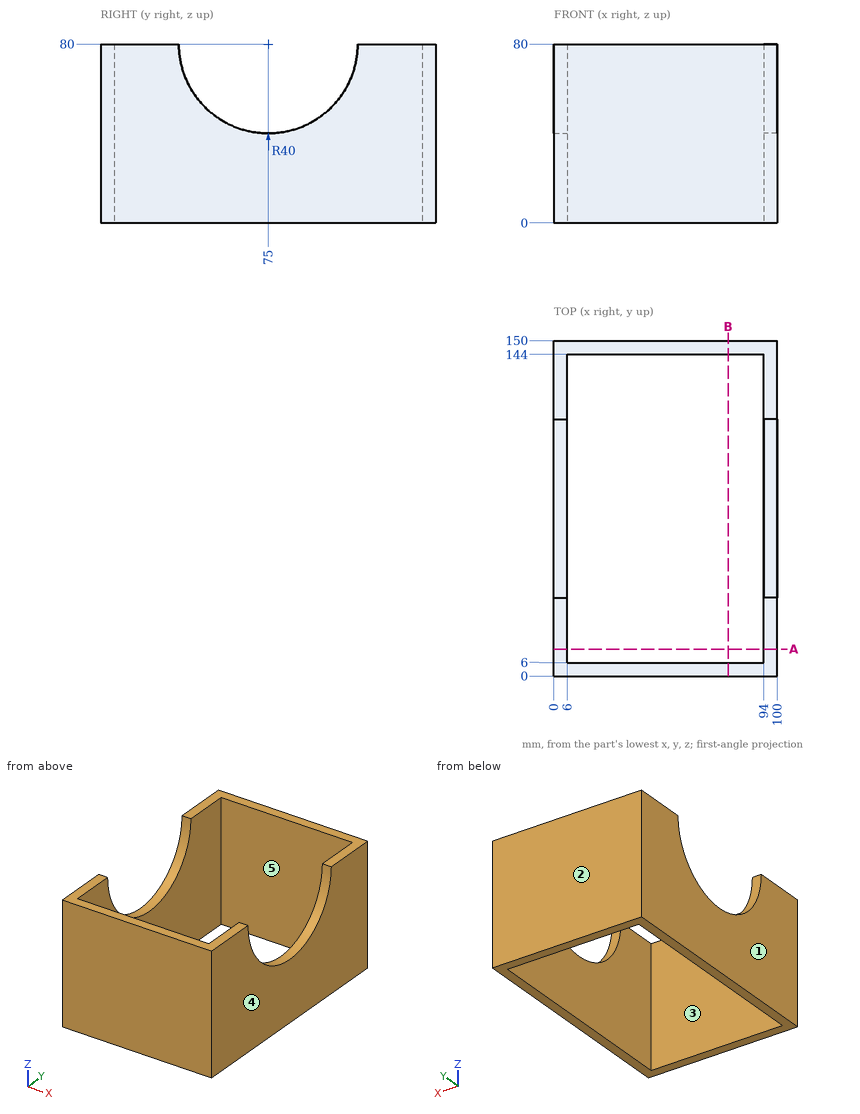
Job drawing, mm, ordinate dimensions from the low corner. One solid piece. A direction names the side the tool comes from. Coordinates: 2 decimals unless noted, no trailing zeros. Loops run counter-clockwise (first coordinate to the right, second up) from the corner with the lowest first, then second, coordinate; pieces in that order, holes last. Notation, with made-up numbers: (-23.75, 2) - (18.25, 2) arc R22 ccw to (18.25, 25) - close; hole circle Ø10 at (26, 73). An arc over 180 degrees is marked (long way). Write item = value, one per line. Start each with the question number.
Q1. Which spindle directions (+Z, -Z, +X, -X, +Y, -Y) get a long thin tool onto all of the face, cutting with end or side? Do the marked faces 4 and 5. Say none if no direction does.
Q2. Drill centre lines: L1, parallel to Y at x = 63.5, z = 9; L2, parallel to X at y = 140.5, z = 11.5. Where is each one in solid material? Low to high.
Q3. Flat gauge pin, fed straight in: pin 1 Ø12 at (x, z) = (43, 23) entering from -Y. Where does the tip first touch, or does it go through?
Q4. Pull direction Y, two halves, no side cores. Call the marked faces 1, 2 and 3: pulls with the +Y half, pulls with the -Y half, needs draft (parallel to the pull), parting line crosses it, or undercut.
Q5. Cut at B-B, the plane x = 78. List the corners of the cut face in (y, z), then the cut area to 3 significant figures.
Q6. Cut at A-A, the plane y = 12. List the corners of the cut face in (x, z).
Computed:
q1.face_4 = +Z, -Z, +X, +Y, -Y
q1.face_5 = +Z, -Z
q2.L1 = 0 to 6, 144 to 150
q2.L2 = 0 to 6, 94 to 100
q3.pin_1 = 0
q4.face_1 = needs draft
q4.face_2 = pulls with the +Y half
q4.face_3 = undercut
q5.outline = (0, 0) - (6, 0) - (6, 80) - (0, 80) - close; (144, 0) - (150, 0) - (150, 80) - (144, 80) - close
q5.area = 960 mm²
q6.outline = (0, 0) - (6, 0) - (6, 80) - (0, 80) - close; (94, 0) - (100, 0) - (100, 80) - (94, 80) - close
